```python
from build123d import *

# Parameters (mm, degrees)
SKETCH1_R           = 9.30275
BOSS_EXTRUDE1_DEPTH = 4.7625
SKETCH1_6_R         = 1.55575
SKETCH1_6_R_2       = 0.762
SKETCH1_6_R_3       = 0.734114047
SKETCH1_6_R_4       = 3.07975
SKETCH1_6_W         = 3.1496
SKETCH1_6_H         = 35.814
SKETCH1_6_W_2       = 23.622
SKETCH1_6_H_2       = 3.1496
CUT_EXTRUDE2_DEPTH  = 4.7625


with BuildPart() as part:
    # Sketch1 → Boss-Extrude1 (new body)
    with BuildSketch(Plane(origin=(0, 0, 0), x_dir=(1, 0, 0), z_dir=(0, 1, 0))):
        with Locations((25.9715, -58.92165)):
            Circle(SKETCH1_R)
        with Locations((-70.4977, 32.16275)):
            Circle(SKETCH1_R)
        with Locations((-70.4977, -32.16275)):
            Circle(SKETCH1_R)
        with Locations((70.4977, 32.16275)):
            Circle(SKETCH1_R)
        with Locations((70.4977, -32.16275)):
            Circle(SKETCH1_R)
        with Locations((25.9715, 58.92165)):
            Circle(SKETCH1_R)
        with Locations((-25.9715, 58.92165)):
            Circle(SKETCH1_R)
        with Locations((-25.9715, -58.92165)):
            Circle(SKETCH1_R)
        Polygon((-75.3872, 32.16275), (-75.3872, -32.16275), (-73.016314747, -36.353667562), (-28.490114747, -63.112567562), (-25.9715, -63.81115), (25.9715, -63.81115), (28.490114747, -63.112567562), (73.016314747, -36.353667562), (75.3872, -32.16275), (75.3872, 32.16275), (73.016314747, 36.353667562), (28.490114747, 63.112567562), (25.9715, 63.81115), (-25.9715, 63.81115), (-28.490114747, 63.112567562), (-73.016314747, 36.353667562), align=None)
    extrude(amount=BOSS_EXTRUDE1_DEPTH)

    # Sketch1_6 → Cut-Extrude2 (cut, symmetric)
    with BuildSketch(Plane(origin=(0, 0, 0), x_dir=(1, 0, 0), z_dir=(0, 1, 0))):
        Polygon((-40.005, -17.907), (-22.4155, -17.907), (-22.4155, -25.019), (22.4155, -25.019), (22.4155, -17.907), (40.005, -17.907), (40.005, 17.907), (22.4155, 17.907), (22.4155, 25.019), (-22.4155, 25.019), (-22.4155, 17.907), (-40.005, 17.907), align=None)
        with Locations(Location((25.45715, -20.94865, 0), (0, 0, 270))):
            Circle(SKETCH1_6_R)
        with Locations(Location((25.45715, 20.94865, 0), (0, 0, 270))):
            Circle(SKETCH1_6_R)
        with Locations(Location((-25.45715, -20.94865, 0), (0, 0, 270))):
            Circle(SKETCH1_6_R)
        with Locations(Location((-25.45715, 20.94865, 0), (0, 0, 270))):
            Circle(SKETCH1_6_R)
        with Locations(Location((71.98995, -37.97935, 0), (0, 0, 270))):
            Circle(SKETCH1_6_R_2)
        with Locations(Location((69.00545, -37.97935, 0), (0, 0, 270))):
            Circle(SKETCH1_6_R_2)
        with Locations(Location((77.1525, -33.9725, 0), (0, 0, 270))):
            Circle(SKETCH1_6_R_2)
        with Locations(Location((77.1525, -30.353, 0), (0, 0, 270))):
            Circle(SKETCH1_6_R_3)
        with Locations(Location((71.98995, -26.34615, 0), (0, 0, 270))):
            Circle(SKETCH1_6_R_2)
        with Locations(Location((69.00545, -26.34615, 0), (0, 0, 270))):
            Circle(SKETCH1_6_R_2)
        with Locations(Location((70.4977, -32.16275, 0), (0, 0, 270))):
            Circle(SKETCH1_6_R_4)
        with Locations(Location((63.8429, -30.353, 0), (0, 0, 270))):
            Circle(SKETCH1_6_R_2)
        with Locations(Location((63.8429, -33.9725, 0), (0, 0, 270))):
            Circle(SKETCH1_6_R_2)
        with Locations((70.4977, 0)):
            Rectangle(SKETCH1_6_W, SKETCH1_6_H)
        with Locations(Location((77.1525, 30.353, 0), (0, 0, 270))):
            Circle(SKETCH1_6_R_2)
        with Locations(Location((77.1525, 33.9725, 0), (0, 0, 270))):
            Circle(SKETCH1_6_R_3)
        with Locations(Location((71.98995, 26.34615, 0), (0, 0, 270))):
            Circle(SKETCH1_6_R_2)
        with Locations(Location((69.00545, 26.34615, 0), (0, 0, 270))):
            Circle(SKETCH1_6_R_2)
        with Locations(Location((70.4977, 32.16275, 0), (0, 0, 270))):
            Circle(SKETCH1_6_R_4)
        with Locations(Location((63.8429, 30.353, 0), (0, 0, 270))):
            Circle(SKETCH1_6_R_2)
        with Locations(Location((63.8429, 33.9725, 0), (0, 0, 270))):
            Circle(SKETCH1_6_R_2)
        with Locations(Location((71.98995, 37.97935, 0), (0, 0, 270))):
            Circle(SKETCH1_6_R_2)
        with Locations(Location((69.00545, 37.97935, 0), (0, 0, 270))):
            Circle(SKETCH1_6_R_2)
        with Locations(Location((32.6263, 57.1119, 0), (0, 0, 270))):
            Circle(SKETCH1_6_R_2)
        with Locations(Location((32.6263, 60.7314, 0), (0, 0, 270))):
            Circle(SKETCH1_6_R_3)
        with Locations(Location((27.46375, 64.73825, 0), (0, 0, 270))):
            Circle(SKETCH1_6_R_2)
        with Locations(Location((24.47925, 64.73825, 0), (0, 0, 270))):
            Circle(SKETCH1_6_R_2)
        with Locations(Location((19.3167, 60.7314, 0), (0, 0, 270))):
            Circle(SKETCH1_6_R_2)
        with Locations(Location((19.3167, 57.1119, 0), (0, 0, 270))):
            Circle(SKETCH1_6_R_2)
        with Locations(Location((24.47925, 53.10505, 0), (0, 0, 270))):
            Circle(SKETCH1_6_R_2)
        with Locations(Location((27.46375, 53.10505, 0), (0, 0, 270))):
            Circle(SKETCH1_6_R_2)
        with Locations(Location((25.9715, 58.92165, 0), (0, 0, 270))):
            Circle(SKETCH1_6_R_4)
        with Locations((0, 58.92165)):
            Rectangle(SKETCH1_6_W_2, SKETCH1_6_H_2)
        with Locations(Location((-19.3167, 57.1119, 0), (0, 0, 270))):
            Circle(SKETCH1_6_R_2)
        with Locations(Location((-19.3167, 60.7314, 0), (0, 0, 270))):
            Circle(SKETCH1_6_R_3)
        with Locations(Location((-24.47925, 64.73825, 0), (0, 0, 270))):
            Circle(SKETCH1_6_R_2)
        with Locations(Location((-27.46375, 64.73825, 0), (0, 0, 270))):
            Circle(SKETCH1_6_R_2)
        with Locations(Location((-32.6263, 60.7314, 0), (0, 0, 270))):
            Circle(SKETCH1_6_R_2)
        with Locations(Location((-32.6263, 57.1119, 0), (0, 0, 270))):
            Circle(SKETCH1_6_R_2)
        with Locations(Location((-27.46375, 53.10505, 0), (0, 0, 270))):
            Circle(SKETCH1_6_R_2)
        with Locations(Location((-24.47925, 53.10505, 0), (0, 0, 270))):
            Circle(SKETCH1_6_R_2)
        with Locations(Location((-25.9715, 58.92165, 0), (0, 0, 270))):
            Circle(SKETCH1_6_R_4)
        with Locations(Location((-69.00545, 37.97935, 0), (0, 0, 270))):
            Circle(SKETCH1_6_R_2)
        with Locations(Location((-71.98995, 37.97935, 0), (0, 0, 270))):
            Circle(SKETCH1_6_R_2)
        with Locations(Location((-77.1525, 33.9725, 0), (0, 0, 270))):
            Circle(SKETCH1_6_R_2)
        with Locations(Location((-77.1525, 30.353, 0), (0, 0, 270))):
            Circle(SKETCH1_6_R_2)
        with Locations(Location((-70.4977, 32.16275, 0), (0, 0, 270))):
            Circle(SKETCH1_6_R_4)
        with Locations(Location((-71.98995, 26.34615, 0), (0, 0, 270))):
            Circle(SKETCH1_6_R_2)
        with Locations(Location((-69.00545, 26.34615, 0), (0, 0, 270))):
            Circle(SKETCH1_6_R_2)
        with Locations(Location((-63.8429, 30.353, 0), (0, 0, 270))):
            Circle(SKETCH1_6_R_2)
        with Locations(Location((-63.8429, 33.9725, 0), (0, 0, 270))):
            Circle(SKETCH1_6_R_3)
        with Locations((-70.4977, 0)):
            Rectangle(SKETCH1_6_W, SKETCH1_6_H)
        with Locations(Location((-69.00545, -26.34615, 0), (0, 0, 270))):
            Circle(SKETCH1_6_R_2)
        with Locations(Location((-71.98995, -26.34615, 0), (0, 0, 270))):
            Circle(SKETCH1_6_R_2)
        with Locations(Location((-77.1525, -30.353, 0), (0, 0, 270))):
            Circle(SKETCH1_6_R_2)
        with Locations(Location((-77.1525, -33.9725, 0), (0, 0, 270))):
            Circle(SKETCH1_6_R_2)
        with Locations(Location((-71.98995, -37.97935, 0), (0, 0, 270))):
            Circle(SKETCH1_6_R_2)
        with Locations(Location((-69.00545, -37.97935, 0), (0, 0, 270))):
            Circle(SKETCH1_6_R_2)
        with Locations(Location((-63.8429, -33.9725, 0), (0, 0, 270))):
            Circle(SKETCH1_6_R_2)
        with Locations(Location((-63.8429, -30.353, 0), (0, 0, 270))):
            Circle(SKETCH1_6_R_3)
        with Locations(Location((-70.4977, -32.16275, 0), (0, 0, 270))):
            Circle(SKETCH1_6_R_4)
        with Locations(Location((-27.46375, -53.10505, 0), (0, 0, 270))):
            Circle(SKETCH1_6_R_2)
        with Locations(Location((-24.47925, -53.10505, 0), (0, 0, 270))):
            Circle(SKETCH1_6_R_2)
        with Locations(Location((-19.3167, -57.1119, 0), (0, 0, 270))):
            Circle(SKETCH1_6_R_3)
        with Locations(Location((-19.3167, -60.7314, 0), (0, 0, 270))):
            Circle(SKETCH1_6_R_2)
        with Locations(Location((-24.47925, -64.73825, 0), (0, 0, 270))):
            Circle(SKETCH1_6_R_2)
        with Locations(Location((-27.46375, -64.73825, 0), (0, 0, 270))):
            Circle(SKETCH1_6_R_2)
        with Locations(Location((-32.6263, -60.7314, 0), (0, 0, 270))):
            Circle(SKETCH1_6_R_2)
        with Locations(Location((-32.6263, -57.1119, 0), (0, 0, 270))):
            Circle(SKETCH1_6_R_2)
        with Locations(Location((-25.9715, -58.92165, 0), (0, 0, 270))):
            Circle(SKETCH1_6_R_4)
        with Locations((0, -58.92165)):
            Rectangle(SKETCH1_6_W_2, SKETCH1_6_H_2)
        with Locations(Location((32.6263, -57.1119, 0), (0, 0, 270))):
            Circle(SKETCH1_6_R_3)
        with Locations(Location((32.6263, -60.7314, 0), (0, 0, 270))):
            Circle(SKETCH1_6_R_2)
        with Locations(Location((27.46375, -64.73825, 0), (0, 0, 270))):
            Circle(SKETCH1_6_R_2)
        with Locations(Location((24.47925, -64.73825, 0), (0, 0, 270))):
            Circle(SKETCH1_6_R_2)
        with Locations(Location((19.3167, -60.7314, 0), (0, 0, 270))):
            Circle(SKETCH1_6_R_2)
        with Locations(Location((19.3167, -57.1119, 0), (0, 0, 270))):
            Circle(SKETCH1_6_R_2)
        with Locations(Location((24.47925, -53.10505, 0), (0, 0, 270))):
            Circle(SKETCH1_6_R_2)
        with Locations(Location((27.46375, -53.10505, 0), (0, 0, 270))):
            Circle(SKETCH1_6_R_2)
        with Locations(Location((25.9715, -58.92165, 0), (0, 0, 270))):
            Circle(SKETCH1_6_R_4)
    extrude(amount=CUT_EXTRUDE2_DEPTH, both=True, mode=Mode.SUBTRACT)


solid = part.part
```
Source: CAD feature listing. Evaluate the final solid. Frame: model axes, mm. A direction names the side the tool comes from. Give positions to 0.01 mm unless a question says otherwise; leave off trailing zeros. Order: outer loops, then holes, each group sorted by start corner. A loop starts at its lowest first (then second) coordinate and runs counter-clockwise, first axis right, second up. Notation, with made-up numbers: (-10, -26.75) -> (46, -26.75) arc R10 cw to (46, -16.75) -> close; hole circle Ø4 at (5.25, 54). An arc over 180 degrees is marked (long way). Use a Markdown table: item, result.
Q1. Access query for faces 1 (the face through (-1, 0, -31)), 2 (the face through (68.923, 2, 0)). Directions: +Z, -Z, +X, -X, +Y, -Y. A direction counts if a zero-diameter tool reaches every point of the face in a straight line with its end or side. Return the directions, or none.
A:
| item | result |
|---|---|
| face 1 | +Z, -Z, +X, -X, -Y |
| face 2 | +Y, -Y |
Q2. Section B-B (y = 1.35). State how many separate pieces and enclosed holes the cut face has, and give its area (3 significant figures).
A:
| item | result |
|---|---|
| separate pieces | 1 |
| enclosed holes | 81 |
| area | 12,800 mm^2 |
Q3. Pull-direction query (X, two-part tool) for faces 3 (the face through (31, 2, 17.907)), 4 (the face through (-1, 4.762, -31)); classes: +X half, -X half, draft (parallel to the pull), parting line (faces both ways), or undercut.
A:
| item | result |
|---|---|
| face 3 | undercut |
| face 4 | draft |
Q4. Section A-A (x = 55). Return the cut outline in (y, z), and give its area (3 significant figures).
A:
| item | result |
|---|---|
| outline | (0, -47.18) -> (4.76, -47.18) -> (4.76, 47.18) -> (0, 47.18) -> close |
| area | 449 mm^2 |
Q5. Section C-C (x = -51). Return the cut outline in (y, z), and give its area (3 significant figures).
A:
| item | result |
|---|---|
| outline | (0, -49.58) -> (4.76, -49.58) -> (4.76, 49.58) -> (0, 49.58) -> close |
| area | 472 mm^2 |
Q6. First-contact query: P1, Ø1.4, axis at y = 2.5, z = -5, coming from the +X side; P2, Ø1.5, axis at y = 1, z = -30, coming from the -X side; P3, Ø1.4, axis at x = -27.46, z = -53.11, coming from the +Y side; P4, Ø1.6, axis at y = 2.5, z = 59, coming from the +X side. Flat tips, straight axial feed; report the tip coordinate or a pass-through.
A:
| item | result |
|---|---|
| P1 | x = 75.39 |
| P2 | x = -79.69 |
| P3 | through |
| P4 | x = 36.66 |
Q7. Material intervals for line 1 (Z direction, x = -11.5, y = 4.3); line 2 (X direction, y = 0.5, z = 6.5) (1 decimal); line 3 (X direction, y = 3.4, z = -32.5), sorted ascending. Write a range as [from, to].
A:
| item | result |
|---|---|
| line 1 | [-63.81, -60.5], [-57.35, -25.02], [25.02, 57.35], [60.5, 63.81] |
| line 2 | [-75.4, -72.1], [-68.9, -40], [40, 68.9], [72.1, 75.4] |
| line 3 | [-79.79, -73.56], [-67.44, 67.44], [73.56, 79.79] |
